```python
from build123d import *

# Parameters (mm, degrees)
SKETCH_W                           = 76.2
SKETCH_H                           = 114.3
PAD_DEPTH                          = 10.16
SKETCH001_R                        = 1.397
HOLE_DEPTH                         = 285.654416
SKETCH002_R                        = 1.905
HOLE001_DEPTH                      = 285.654416
SKETCH001_MIRRORED_2_R             = 1.397
HOLE_MIRRORED_2_DEPTH              = 285.654416
SKETCH002_LINEARPATTERN_2_R        = 1.905
HOLE001_LINEARPATTERN_2_DEPTH      = 285.654416
SKETCH002_LINEARPATTERN_3_R        = 1.905
HOLE001_LINEARPATTERN_3_DEPTH      = 285.654416
SKETCH002_LINEARPATTERN_4_R        = 1.905
HOLE001_LINEARPATTERN_4_DEPTH      = 285.654416
SKETCH002_LINEARPATTERN_5_R        = 1.905
HOLE001_LINEARPATTERN_5_DEPTH      = 285.654416
SKETCH002_LINEARPATTERN_6_R        = 1.905
HOLE001_LINEARPATTERN_6_DEPTH      = 285.654416
SKETCH003_W                        = 50.8
SKETCH003_H                        = 88.9
POCKET_DEPTH                       = 2.54
SKETCH004_R                        = 2.54
HOLE002_DEPTH                      = 285.654416
SKETCH004_MIRRORED003_2_R          = 2.54
HOLE002_MIRRORED003_2_DEPTH        = 285.654416
POCKET001_DEPTH                    = 2.921
POCKET001_LINEARPATTERN001_2_DEPTH = 2.921
POCKET001_LINEARPATTERN001_3_DEPTH = 2.921
POCKET001_LINEARPATTERN001_4_DEPTH = 2.921
POCKET001_LINEARPATTERN001_5_DEPTH = 2.921
POCKET001_LINEARPATTERN001_6_DEPTH = 2.921


with BuildPart() as part:
    # Sketch → Pad (new body)
    with BuildSketch(Plane.XY):
        Rectangle(SKETCH_W, SKETCH_H)
    extrude(amount=PAD_DEPTH)

    # Sketch001 (on Face6 of Pad) → Hole (cut, through all)
    with BuildSketch(Plane.XY.offset(10.16)):
        with Locations((-31.75, 40.64)):
            Circle(SKETCH001_R)
    hole = extrude(amount=-HOLE_DEPTH, mode=Mode.SUBTRACT)

    # Sketch002 (on Face5 of Hole) → Hole001 (cut, through all)
    with BuildSketch(Plane.XY.offset(10.16)):
        with Locations((-31.75, 33.02)):
            Circle(SKETCH002_R)
    hole001 = extrude(amount=-HOLE001_DEPTH, mode=Mode.SUBTRACT)

    # Sketch001 Mirrored 2 → Hole Mirrored 2 (cut, through all)
    with BuildSketch(Plane(origin=(0, 0, 10.16), x_dir=(-1, 0, 0), z_dir=(0, 0, -1))):
        with Locations((-31.75, 40.64)):
            Circle(SKETCH001_MIRRORED_2_R)
    hole_mirrored_2 = extrude(amount=HOLE_MIRRORED_2_DEPTH, mode=Mode.SUBTRACT)

    # Mirrored001: Hole, Hole Mirrored 2 across Sketch001 H_Axis
    add(hole.mirror(Plane(origin=(0, 0, 10.16), x_dir=(0, 0, 1), z_dir=(0, 1, 0))), mode=Mode.SUBTRACT)
    add(hole_mirrored_2.mirror(Plane(origin=(0, 0, 10.16), x_dir=(0, 0, 1), z_dir=(0, 1, 0))), mode=Mode.SUBTRACT)

    # Sketch002 LinearPattern 2 → Hole001 LinearPattern 2 (cut, through all)
    with BuildSketch(Plane(origin=(0, -12.7, 10.16), x_dir=(1, 0, 0), z_dir=(0, 0, 1))):
        with Locations((-31.75, 33.02)):
            Circle(SKETCH002_LINEARPATTERN_2_R)
    hole001_linearpattern_2 = extrude(amount=-HOLE001_LINEARPATTERN_2_DEPTH, mode=Mode.SUBTRACT)

    # Sketch002 LinearPattern 3 → Hole001 LinearPattern 3 (cut, through all)
    with BuildSketch(Plane(origin=(0, -25.4, 10.16), x_dir=(1, 0, 0), z_dir=(0, 0, 1))):
        with Locations((-31.75, 33.02)):
            Circle(SKETCH002_LINEARPATTERN_3_R)
    hole001_linearpattern_3 = extrude(amount=-HOLE001_LINEARPATTERN_3_DEPTH, mode=Mode.SUBTRACT)

    # Sketch002 LinearPattern 4 → Hole001 LinearPattern 4 (cut, through all)
    with BuildSketch(Plane(origin=(0, -38.1, 10.16), x_dir=(1, 0, 0), z_dir=(0, 0, 1))):
        with Locations((-31.75, 33.02)):
            Circle(SKETCH002_LINEARPATTERN_4_R)
    hole001_linearpattern_4 = extrude(amount=-HOLE001_LINEARPATTERN_4_DEPTH, mode=Mode.SUBTRACT)

    # Sketch002 LinearPattern 5 → Hole001 LinearPattern 5 (cut, through all)
    with BuildSketch(Plane(origin=(0, -50.8, 10.16), x_dir=(1, 0, 0), z_dir=(0, 0, 1))):
        with Locations((-31.75, 33.02)):
            Circle(SKETCH002_LINEARPATTERN_5_R)
    hole001_linearpattern_5 = extrude(amount=-HOLE001_LINEARPATTERN_5_DEPTH, mode=Mode.SUBTRACT)

    # Sketch002 LinearPattern 6 → Hole001 LinearPattern 6 (cut, through all)
    with BuildSketch(Plane(origin=(0, -63.5, 10.16), x_dir=(1, 0, 0), z_dir=(0, 0, 1))):
        with Locations((-31.75, 33.02)):
            Circle(SKETCH002_LINEARPATTERN_6_R)
    hole001_linearpattern_6 = extrude(amount=-HOLE001_LINEARPATTERN_6_DEPTH, mode=Mode.SUBTRACT)

    # Mirrored002: Hole001, Hole001 LinearPattern 2, Hole001 LinearPattern 3, Hole001 LinearPattern 4, Hole001 LinearPattern 5, Hole001 LinearPattern 6 across Sketch002 V_Axis
    add(hole001.mirror(Plane(origin=(0, 0, 10.16), x_dir=(0, 0, 1), z_dir=(1, 0, 0))), mode=Mode.SUBTRACT)
    add(hole001_linearpattern_2.mirror(Plane(origin=(0, 0, 10.16), x_dir=(0, 0, 1), z_dir=(1, 0, 0))), mode=Mode.SUBTRACT)
    add(hole001_linearpattern_3.mirror(Plane(origin=(0, 0, 10.16), x_dir=(0, 0, 1), z_dir=(1, 0, 0))), mode=Mode.SUBTRACT)
    add(hole001_linearpattern_4.mirror(Plane(origin=(0, 0, 10.16), x_dir=(0, 0, 1), z_dir=(1, 0, 0))), mode=Mode.SUBTRACT)
    add(hole001_linearpattern_5.mirror(Plane(origin=(0, 0, 10.16), x_dir=(0, 0, 1), z_dir=(1, 0, 0))), mode=Mode.SUBTRACT)
    add(hole001_linearpattern_6.mirror(Plane(origin=(0, 0, 10.16), x_dir=(0, 0, 1), z_dir=(1, 0, 0))), mode=Mode.SUBTRACT)

    # Sketch003 (on Face5 of MultiTransform001) → Pocket (cut)
    with BuildSketch(Plane.XY.offset(10.16)):
        Rectangle(SKETCH003_W, SKETCH003_H)
    extrude(amount=-POCKET_DEPTH, mode=Mode.SUBTRACT)

    # Sketch004 (on Face5 of Pocket) → Hole002 (cut, through all)
    with BuildSketch(Plane.XY.offset(10.16)):
        with Locations((-31.75, 50.8)):
            Circle(SKETCH004_R)
    hole002 = extrude(amount=-HOLE002_DEPTH, mode=Mode.SUBTRACT)

    # Sketch004 Mirrored003 2 → Hole002 Mirrored003 2 (cut, through all)
    with BuildSketch(Plane(origin=(0, 0, 10.16), x_dir=(-1, 0, 0), z_dir=(0, 0, -1))):
        with Locations((-31.75, 50.8)):
            Circle(SKETCH004_MIRRORED003_2_R)
    hole002_mirrored003_2 = extrude(amount=HOLE002_MIRRORED003_2_DEPTH, mode=Mode.SUBTRACT)

    # Mirrored004: Hole002, Hole002 Mirrored003 2 across Sketch004 H_Axis
    add(hole002.mirror(Plane(origin=(0, 0, 10.16), x_dir=(0, 0, 1), z_dir=(0, 1, 0))), mode=Mode.SUBTRACT)
    add(hole002_mirrored003_2.mirror(Plane(origin=(0, 0, 10.16), x_dir=(0, 0, 1), z_dir=(0, 1, 0))), mode=Mode.SUBTRACT)

    # Sketch005 (on Face5 of MultiTransform002) → Pocket001 (cut)
    with BuildSketch(Plane.XY.offset(10.16)):
        Polygon((-29.21, 37.419409), (-34.29, 37.419409), (-36.83, 33.02), (-34.29, 28.620591), (-29.21, 28.620591), (-26.67, 33.02), align=None)
    pocket001 = extrude(amount=-POCKET001_DEPTH, mode=Mode.SUBTRACT)

    # Sketch005 LinearPattern001 2 → Pocket001 LinearPattern001 2 (cut)
    with BuildSketch(Plane(origin=(0, -12.7, 10.16), x_dir=(1, 0, 0), z_dir=(0, 0, 1))):
        Polygon((-29.21, 37.419409), (-34.29, 37.419409), (-36.83, 33.02), (-34.29, 28.620591), (-29.21, 28.620591), (-26.67, 33.02), align=None)
    pocket001_linearpattern001_2 = extrude(amount=-POCKET001_LINEARPATTERN001_2_DEPTH, mode=Mode.SUBTRACT)

    # Sketch005 LinearPattern001 3 → Pocket001 LinearPattern001 3 (cut)
    with BuildSketch(Plane(origin=(0, -25.4, 10.16), x_dir=(1, 0, 0), z_dir=(0, 0, 1))):
        Polygon((-29.21, 37.419409), (-34.29, 37.419409), (-36.83, 33.02), (-34.29, 28.620591), (-29.21, 28.620591), (-26.67, 33.02), align=None)
    pocket001_linearpattern001_3 = extrude(amount=-POCKET001_LINEARPATTERN001_3_DEPTH, mode=Mode.SUBTRACT)

    # Sketch005 LinearPattern001 4 → Pocket001 LinearPattern001 4 (cut)
    with BuildSketch(Plane(origin=(0, -38.1, 10.16), x_dir=(1, 0, 0), z_dir=(0, 0, 1))):
        Polygon((-29.21, 37.419409), (-34.29, 37.419409), (-36.83, 33.02), (-34.29, 28.620591), (-29.21, 28.620591), (-26.67, 33.02), align=None)
    pocket001_linearpattern001_4 = extrude(amount=-POCKET001_LINEARPATTERN001_4_DEPTH, mode=Mode.SUBTRACT)

    # Sketch005 LinearPattern001 5 → Pocket001 LinearPattern001 5 (cut)
    with BuildSketch(Plane(origin=(0, -50.8, 10.16), x_dir=(1, 0, 0), z_dir=(0, 0, 1))):
        Polygon((-29.21, 37.419409), (-34.29, 37.419409), (-36.83, 33.02), (-34.29, 28.620591), (-29.21, 28.620591), (-26.67, 33.02), align=None)
    pocket001_linearpattern001_5 = extrude(amount=-POCKET001_LINEARPATTERN001_5_DEPTH, mode=Mode.SUBTRACT)

    # Sketch005 LinearPattern001 6 → Pocket001 LinearPattern001 6 (cut)
    with BuildSketch(Plane(origin=(0, -63.5, 10.16), x_dir=(1, 0, 0), z_dir=(0, 0, 1))):
        Polygon((-29.21, 37.419409), (-34.29, 37.419409), (-36.83, 33.02), (-34.29, 28.620591), (-29.21, 28.620591), (-26.67, 33.02), align=None)
    pocket001_linearpattern001_6 = extrude(amount=-POCKET001_LINEARPATTERN001_6_DEPTH, mode=Mode.SUBTRACT)

    # Mirrored005: Pocket001, Pocket001 LinearPattern001 2, Pocket001 LinearPattern001 3, Pocket001 LinearPattern001 4, Pocket001 LinearPattern001 5, Pocket001 LinearPattern001 6 across Sketch005 V_Axis
    add(pocket001.mirror(Plane(origin=(0, 0, 10.16), x_dir=(0, 0, 1), z_dir=(1, 0, 0))), mode=Mode.SUBTRACT)
    add(pocket001_linearpattern001_2.mirror(Plane(origin=(0, 0, 10.16), x_dir=(0, 0, 1), z_dir=(1, 0, 0))), mode=Mode.SUBTRACT)
    add(pocket001_linearpattern001_3.mirror(Plane(origin=(0, 0, 10.16), x_dir=(0, 0, 1), z_dir=(1, 0, 0))), mode=Mode.SUBTRACT)
    add(pocket001_linearpattern001_4.mirror(Plane(origin=(0, 0, 10.16), x_dir=(0, 0, 1), z_dir=(1, 0, 0))), mode=Mode.SUBTRACT)
    add(pocket001_linearpattern001_5.mirror(Plane(origin=(0, 0, 10.16), x_dir=(0, 0, 1), z_dir=(1, 0, 0))), mode=Mode.SUBTRACT)
    add(pocket001_linearpattern001_6.mirror(Plane(origin=(0, 0, 10.16), x_dir=(0, 0, 1), z_dir=(1, 0, 0))), mode=Mode.SUBTRACT)


solid = part.part
```
Source: CAD feature listing. Evaluate the final solid. Frame: model axes, mm. Round coordinates to 2 decimals unless told otherwise and drop trailing zeros. Loops run counter-clockwise (first coordinate to the right, second up) from the corner with the lowest first, then second, coordinate; pieces in that order, holes last.
1. Contact query for flat-ended pins moving along their axis: pin 1 (9.5 mm diameter, centred on x = 31, y = -31, fed in from +Z); pin 2 (4.5 mm diameter, centred on x = 31.5, y = 8, fed in from +Z). Output: stop coordinate, or through.
2. Section query C-C on x = 21.5. Output: boundary loops of the cut face in (y, z), and give its area (3 significant figures).
3. Section query B-B on z = 3.75. Give the number of separate pieces and of enclosed holes in the cut face, and give its area (3 significant figures).
4. Section query A-A on y = 50.8. Output: boundary loops of the cut face in (x, z), and give its area (3 significant figures).
5. Section query D-D on y = -38. Output: boundary loops of the cut face in (x, z), and give its area (3 significant figures).
6. Ray query, L1, parallel to Y at x = -25, z = 9; L2, parallel to X at y = 26, z = 7.75; L3, parallel to X at y = -41.5, z = 7. Return the intervals inside material, ascending.
7. Mould query, pull axis X, two halves, no side actions, for faces 1 (the flat face through (-1, 57.15, 5)), 2 (the flat face through (27.958, -32.711, 8.72)). Classes: released by +X, released by -X, zero draft, split by the parting line, or undercut.
Answers below:
1. pin 1: stops at z = 10.16
1. pin 2: stops at z = 7.24
2. outline: (-57.15, 0) - (57.15, 0) - (57.15, 10.16) - (44.45, 10.16) - (44.45, 7.62) - (-44.45, 7.62) - (-44.45, 10.16) - (-57.15, 10.16) - close
2. area: 935 mm2
3. separate pieces: 1
3. enclosed holes: 20
3. area: 8,470 mm2
4. outline: (-38.1, 0) - (-34.29, 0) - (-34.29, 10.16) - (-38.1, 10.16) - close; (-29.21, 0) - (29.21, 0) - (29.21, 10.16) - (-29.21, 10.16) - close; (34.29, 0) - (38.1, 0) - (38.1, 10.16) - (34.29, 10.16) - close
4. area: 671 mm2
5. outline: (-38.1, 0) - (38.1, 0) - (38.1, 10.16) - (25.4, 10.16) - (25.4, 7.62) - (-25.4, 7.62) - (-25.4, 10.16) - (-38.1, 10.16) - close
5. area: 645 mm2
6. L1: y = -57.15 to -44.45, 44.45 to 57.15
6. L2: x = -38.1 to -25.4, 25.4 to 38.1
6. L3: x = -38.1 to -32.85, -30.65 to 30.65, 32.85 to 38.1
7. face 1: zero draft
7. face 2: undercut
